Could you check a few things on this drawing? It's one solid part, dimensions in mm from its lowest x, y, z. Give positions to 0.01 mm unless a question says otherwise; leave off trailing zeros. Order: outer loops, then holes, each group sorted by start corner. A loop starts at its lowest first (then second) coordinate and runs counter-clockwise, first axis right, second up.
(1) Imagine slicing it at B-B, the plane y = 4. State how many separate pieces and enclosed holes the cut face has, then the cut area to 4 significant figures.
(2) Will these pins go through, and if not, where does the flat tip stop? pin 1 (3 mm diameter, centred on x = 4, z = 3.5, fed in from +Y); pin 2 (2.5 mm diameter, centred on x = 5, z = 4, fed in from -Y).
(3) If I drill on probe 1 along Z at (x, y) = (4, 0.3); probe 2 along Z at (x, y) = (5.75, 1.65); probe 3 along X at (y, z) = (5.2, 76.5), over which ranges is the centre line in solid material (lowest first)?
(4) Imagine slicing it at A-A, the plane x = 5. Write out the boundary of the cut face in (y, z).
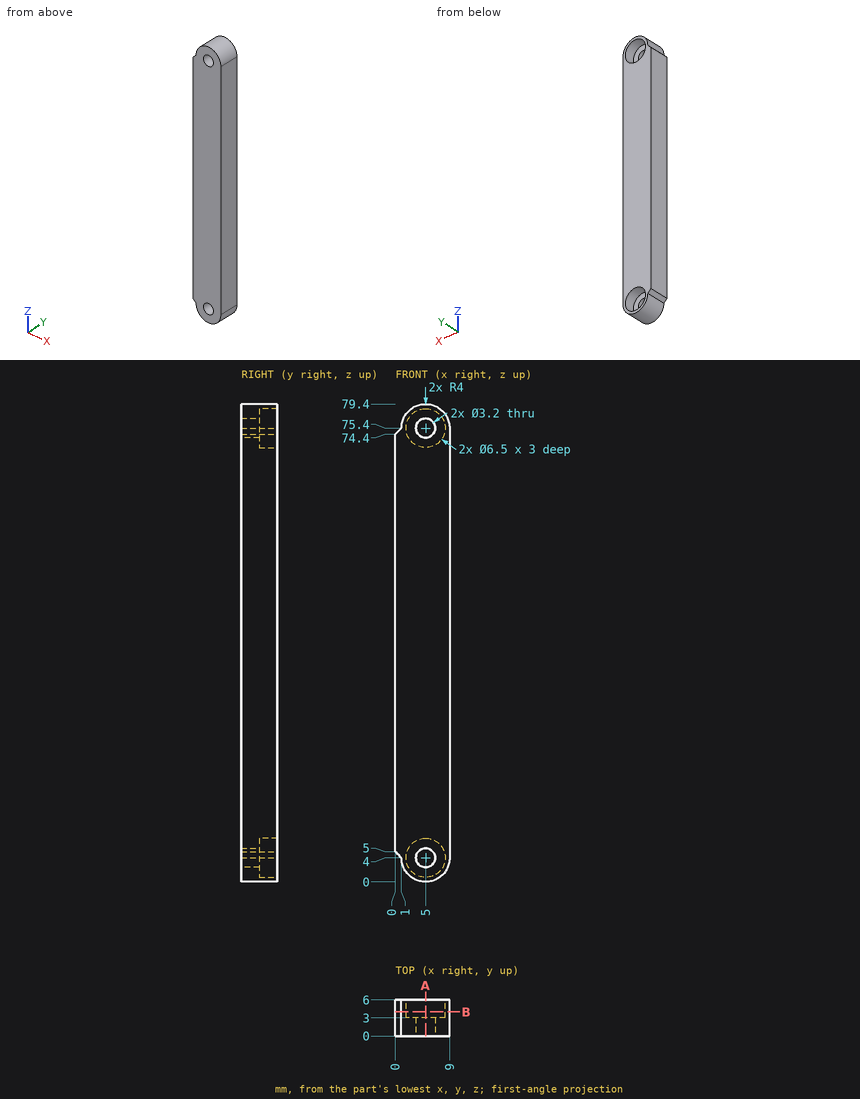
Answer block:
1. separate pieces: 1
1. enclosed holes: 2
1. area: 625.5 mm2
2. pin 1: stops at y = 3
2. pin 2: passes through
3. probe 1: z = 0.13 to 2.75, 5.25 to 74.15, 76.65 to 79.27
3. probe 2: z = 0.07 to 2.59, 5.41 to 73.99, 76.81 to 79.33
3. probe 3: x = 1.15 to 1.94, 8.06 to 8.85
4. outline: (0, 0) - (6, 0) - (6, 0.75) - (3, 0.75) - (3, 2.4) - (0, 2.4) - close; (0, 5.6) - (3, 5.6) - (3, 7.25) - (6, 7.25) - (6, 72.15) - (3, 72.15) - (3, 73.8) - (0, 73.8) - close; (0, 77) - (3, 77) - (3, 78.65) - (6, 78.65) - (6, 79.4) - (0, 79.4) - close
